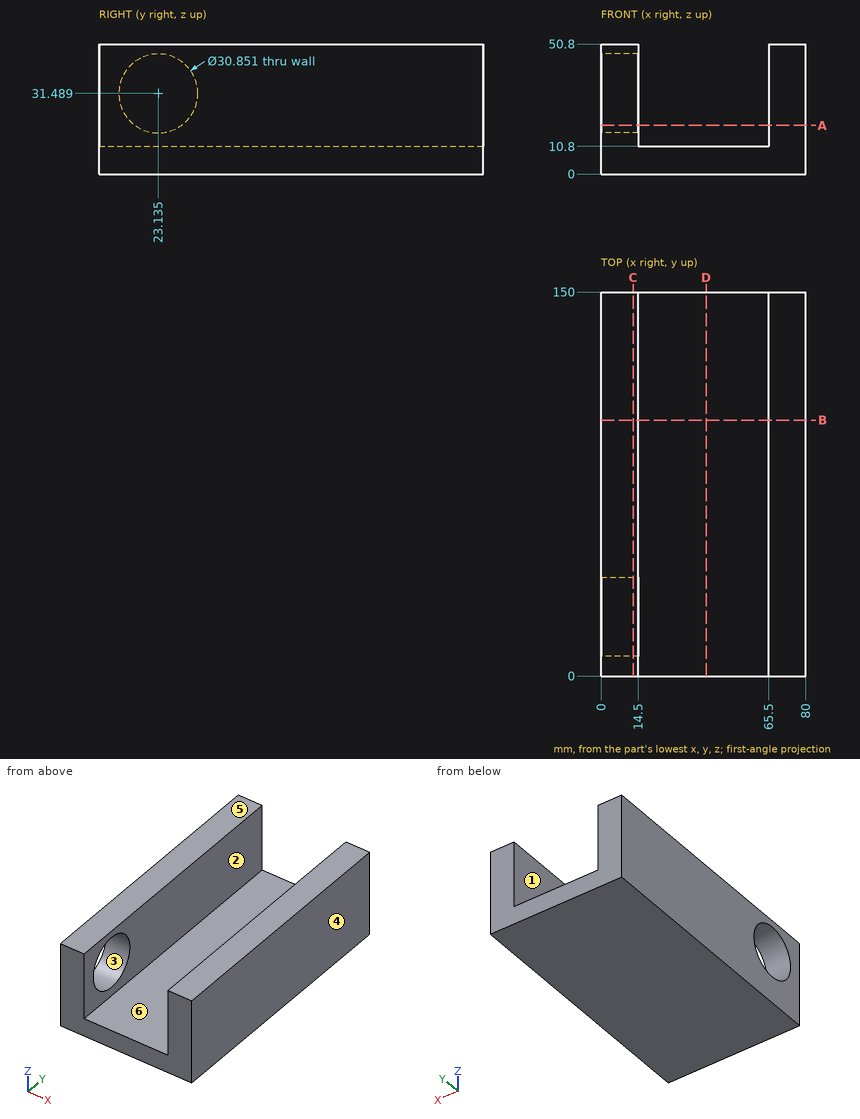
Here's the drawing with two shaded views (mm, measured from the low corner). I have some questions. A direction names the side the tool comes from. Round coordinates to 2 decimals unless told otherwise and drop trailing zeros. Order: outer loops, then holes, each group sorted by start corner. A loop starts at its lowest first (then second) coordinate and runs counter-clockwise, first axis right, second up. Notation, with made-up numbers: (42, 7) -> (94, 7) arc R26 ccw to (94, 23) -> close; hole circle Ø11 at (-3.75, 66). An arc over 180 degrees is marked (long way). Return JSON: item names as keys, results as strings.
Q1. For pin 1 Ø10 at (x, z) = (27, 14) entering from -Y; pin 2 Ø15.5 at (x, y) = (35, 84) entering from +Z, each with a flat end and sliding along its axis, tell me the tip position at first contact or that it passes through.
Filled sheet:
{"pin 1": "stops at y = 0", "pin 2": "stops at z = 10.8"}
Q2. If we mould it in two halves opening along X, with no side actions, what happens to the marked faces 1, 2, 3 and 4? For each: released by +X, released by -X, zero draft, split by the parting line, or undercut.
Filled sheet:
{"face 1": "undercut", "face 2": "undercut", "face 3": "zero draft", "face 4": "released by +X"}
Q3. If we section it at D-D on x = 41: List the corners of the cut face in (y, z) for me.
Filled sheet:
{"outline": "(0, 0) -> (150, 0) -> (150, 10.8) -> (0, 10.8) -> close"}
Q4. If we section it at A-A on z = 19: List the corners of the cut face in (x, y) for me, plus the area to 3 significant figures.
Filled sheet:
{"outline": "(0, 0) -> (14.5, 0) -> (14.5, 14.08) -> (0, 14.08) -> close; (0, 32.19) -> (14.5, 32.19) -> (14.5, 150) -> (0, 150) -> close; (65.5, 0) -> (80, 0) -> (80, 150) -> (65.5, 150) -> close", "area": "4,090 mm^2"}
Q5. If we section it at B-B on y = 100: List the corners of the cut face in (x, z) for me, plus the area to 3 significant figures.
Filled sheet:
{"outline": "(0, 0) -> (80, 0) -> (80, 50.8) -> (65.5, 50.8) -> (65.5, 10.8) -> (14.5, 10.8) -> (14.5, 50.8) -> (0, 50.8) -> close", "area": "2,020 mm^2"}
Q6. Which directions (+Z, -Z, +X, -X, +Y, -Y) give clear straight access to the entire face, cutting with the end or side of a thin tool? Please do the marked faces 5 and 6.
Filled sheet:
{"face 5": "+Z, +X, -X, +Y, -Y", "face 6": "+Z, +Y, -Y"}
Q7. I need wall thicknesses on line 1 along X through (y, z) = (26, 14.5); line 2 along Z through (x, y) = (15, 137); line 3 along X through (y, z) = (29, 41). Which ranges of each line are inside material? Lowest first, please. Write a range as from..to.
Filled sheet:
{"line 1": "x = 0..14.5, 65.5..80", "line 2": "z = 0..10.8", "line 3": "x = 65.5..80"}
Q8. If we section it at C-C on x = 12.5: List the corners of the cut face in (y, z) for me (1 decimal).
Filled sheet:
{"outline": "(0, 0) -> (150, 0) -> (150, 50.8) -> (0, 50.8) -> close; hole circle Ø30.9 at (23.1, 31.5)"}
